Could you check a few things on this model? Use its own coordinates, in mm. Face numbers are marked on the shaded views. A direction names the side the tool comes from. Round coordinates to 2 decimals unless told otherwise and drop trailing zeros. Loops run counter-clockwise (first coordinate to the right, second up) from the corner with the lowest first, then second, coordinate; pieces in that order, holes last.
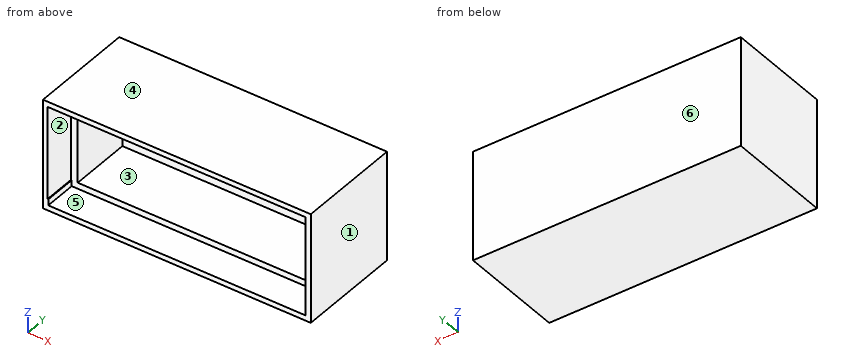
from build123d import *

# Parameters (mm, degrees)
F1_DEPTH = 23
F3_DEPTH = 3
F5_DEPTH = 1.6
F7_DEPTH = 3
F9_DEPTH = 1.6


with BuildPart() as f1:
    # F0 (on Top) → F1 (new body)
    with BuildSketch(Plane.XY):
        Polygon((-65, 25), (0, 25), (0, 8.6), (1.6, 8.6), (1.6, 0), (3, 0), (3, 28), (-68, 28), (-68, 0), (-66.8, 0), (-66.8, 8.6), (-65, 8.6), align=None)
    extrude(amount=F1_DEPTH)

    # F2 (on face) → F3 (join)
    with BuildSketch(Plane.XY.offset(23)):
        Polygon((3, 28), (-68, 28), (-68, 0), (-66.8, 0), (-66.8, 8.6), (-65, 8.6), (-65, 25), (0, 25), (0, 8.6), (1.6, 8.6), (1.6, 0), (3, 0), align=None)
        Polygon((-66.8, 8.6), (-66.8, 0), (1.6, 0), (1.6, 8.6), (0, 8.6), (0, 25), (-65, 25), (-65, 8.6), align=None)
    extrude(amount=F3_DEPTH)

    # F4 (on face) → F5 (cut)
    with BuildSketch(Plane(origin=(0, 0, 23), x_dir=(1, 0, 0), z_dir=(0, 0, -1))):
        Polygon((1.6, 0), (-66.8, 0), (-66.8, -8.6), (-65, -8.6), (0, -8.6), (1.6, -8.6), align=None)
    extrude(amount=-F5_DEPTH, mode=Mode.SUBTRACT)

    # F6 (on face) → F7 (join)
    with BuildSketch(Plane(origin=(0, 0, 0), x_dir=(1, 0, 0), z_dir=(0, 0, -1))):
        Polygon((-66.8, 0), (-68, 0), (-68, -28), (3, -28), (3, 0), (1.6, 0), (1.6, -8.6), (0, -8.6), (0, -25), (-65, -25), (-65, -8.6), (-66.8, -8.6), align=None)
        Polygon((1.6, 0), (-66.8, 0), (-66.8, -8.6), (-65, -8.6), (-65, -25), (0, -25), (0, -8.6), (1.6, -8.6), align=None)
    extrude(amount=F7_DEPTH)

    # F8 (on face) → F9 (cut)
    with BuildSketch(Plane.XY):
        Polygon((-65, 8.6), (-66.6, 8.6), (-66.6, 0), (1.6, 0), (1.6, 8.6), (0, 8.6), align=None)
    extrude(amount=-F9_DEPTH, mode=Mode.SUBTRACT)


solid = f1.part
Item 1: If we section it at C-C, the plane x = -15: Please give me the cut outline in (y, z).
Results list:
outline: (0, -3) - (28, -3) - (28, 26) - (0, 26) - (0, 24.6) - (8.6, 24.6) - (8.6, 23) - (25, 23) - (25, 0) - (8.6, 0) - (8.6, -1.6) - (0, -1.6) - close
Item 2: If I drill on line 1 along Z through (x, y) = (-35, 20); line 2 along X through (y, z) = (23.5, 12.5); line 3 along Z through (x, y) = (-26, 6.75), over which ranges is the centre line in solid material (lowest first)?
Results list:
line 1: z = -3 to 0, 23 to 26
line 2: x = -68 to -65, 0 to 3
line 3: z = -3 to -1.6, 24.6 to 26
Item 3: Will this pin go through, and if not, where does the flat tip stop? pin 1 (1.5 mm diameter, centred on x = -37.5, z = 7, fed in from -Y).
Results list:
pin 1: stops at y = 25
Item 4: For the marked faces 5 and 6, which set-ups out of +Z, -Z, +X, -X, +Y, -Y let a thin tool reach every point of the face, with its end or its side?
Results list:
face 5: -Y
face 6: +Z, -Z, +X, -X, +Y
Item 5: If we section it at B-B, the plane z = 5.75: Please give me the cut outline in (x, y).
Results list:
outline: (-68, 0) - (-66.8, 0) - (-66.8, 8.6) - (-65, 8.6) - (-65, 25) - (0, 25) - (0, 8.6) - (1.6, 8.6) - (1.6, 0) - (3, 0) - (3, 28) - (-68, 28) - close
Item 6: We'd pull the mould along X, two halves only. Please class the marked faces 1, 2, 3 and 4: released by +X, released by -X, zero draft, split by the parting line, or undercut.
Results list:
face 1: released by +X
face 2: undercut
face 3: undercut
face 4: zero draft
Item 7: If we section it at A-A, the plane y = 13.5: Please give me the cut outline in (x, z), then the cut area to 3 significant figures.
Results list:
outline: (-68, -3) - (3, -3) - (3, 26) - (-68, 26) - close; hole (-65, 0) - (0, 0) - (0, 23) - (-65, 23) - close
area: 564 mm2
